Design review of the part built by this model. Coordinates are the model's own, in mm. A direction names the side the tool comes from. Round coordinates to 2 decimals unless told otherwise and drop trailing zeros. Write each loop counter-clockwise with the first axis right and the second up, starting at its lowest first coordinate (ties: lowest second). Pieces come first, ordered by that corner, then holes. Notation, with made-up numbers: (58, 82) -> (73, 82) arc R14 ccw to (73, 95) -> close; hole circle Ø8 at (-0.75, -11.75). An arc over 180 degrees is marked (long way). One line per question, with ' | ' between items. Start each with the question number.
1) For faces 1 (the flat face through (108.839, 0, 3)), 2 (the cylindrical face through (28.573, 0.209, 3.131)), 3 (the cylindrical face through (98.007, 1.411, 2.88)), list the 3-axis set-ups (+Z, -Z, +X, -X, +Y, -Y) from which the entire face can be reached by the end or side of a thin tool; tool diameter is ignored.
2) For probe 1 along Y at (x, z) = (-4.5, 1.5) (3 decimals); probe 2 along X at (y, z) = (2.5, 5); probe 3 along Y at (x, z) = (22, 2.25), list the stretches that pass through material, from the lowest coordinate up.
3) Insertion check: pin 1 Ø1 at (x, y) = (-29, 24.5) entering from -Z; pin 2 Ø3 at (x, y) = (101.5, -0.5) entering from -Z. Each pin has a flat end and moves straight along its axis. Give the tip position at first contact, or say it passes through.
4) Consider section B-B (z = 4.5). Give the boundary of the cut face in (x, y) (3 decimals).
5) Consider section A-A (y = 0). Give the boundary of the cut face in (x, z) (3 decimals), then the cut area to 3 significant figures.
```python
from build123d import *

# Parameters (mm, degrees)
SKETCH1_W               = 217.678
SKETCH1_H               = 63.5
BOSS_EXTRUDE1_DEPTH     = 6.35
CUT_EXTRUDE1_DEPTH      = 114.553128187
CUT_EXTRUDE1_DEPTH_BACK = 114.553128187
SKETCH3_R               = 4.699
CUT_EXTRUDE2_DEPTH      = 5.842


with BuildPart() as part:
    # Sketch1 → Boss-Extrude1 (new body)
    with BuildSketch(Plane.XY):
        Rectangle(SKETCH1_W, SKETCH1_H)
    extrude(amount=BOSS_EXTRUDE1_DEPTH)

    # Sketch2 → Cut-Extrude1 (cut, two sides: drawn at the far end of the back side and taken through both)
    with BuildSketch(Plane.XY.offset(6.35).offset(-CUT_EXTRUDE1_DEPTH_BACK)):
        with BuildLine():
            Line((19.05, -9.525), (-19.05, -9.525))
            ThreePointArc((-19.05, -9.525), (-28.575, 0), (-19.05, 9.525))
            Line((-19.05, 9.525), (19.05, 9.525))
            ThreePointArc((19.05, 9.525), (28.575, 0), (19.05, -9.525))
        make_face()
    extrude(amount=CUT_EXTRUDE1_DEPTH + CUT_EXTRUDE1_DEPTH_BACK, mode=Mode.SUBTRACT)

    # Sketch3 → Cut-Extrude2 (cut)
    with BuildSketch(Plane(origin=(0, 0, 0), x_dir=(-1, 0, 0), z_dir=(0, 0, -1))):
        with Locations((-102.489, 0)):
            Circle(SKETCH3_R)
        with Locations((102.489, 0)):
            Circle(SKETCH3_R)
    extrude(amount=-CUT_EXTRUDE2_DEPTH, mode=Mode.SUBTRACT)


solid = part.part
```
From the geometry:
1) face 1: +Z, -Z, +X, +Y, -Y | face 2: +Z, -Z | face 3: -Z
2) probe 1: y = -31.75 to -9.525, 9.525 to 31.75 | probe 2: x = -108.84 to -106.47, -98.51 to -28.24, 28.24 to 98.51, 106.47 to 108.84 | probe 3: y = -31.75 to -9.06, 9.06 to 31.75
3) pin 1: stops at z = 0 | pin 2: stops at z = 5.84
4) outline: (-108.839, -31.75) -> (108.839, -31.75) -> (108.839, 31.75) -> (-108.839, 31.75) -> close; hole circle Ø9.398 at (-102.489, 0); hole (-19.05, -9.525) -> (19.05, -9.525) arc R9.525 ccw to (19.05, 9.525) -> (-19.05, 9.525) arc R9.525 ccw to start; hole circle Ø9.398 at (102.489, 0)
5) outline: (-108.839, 0) -> (-107.188, 0) -> (-107.188, 5.842) -> (-97.79, 5.842) -> (-97.79, 0) -> (-28.575, 0) -> (-28.575, 6.35) -> (-108.839, 6.35) -> close; (28.575, 0) -> (97.79, 0) -> (97.79, 5.842) -> (107.188, 5.842) -> (107.188, 0) -> (108.839, 0) -> (108.839, 6.35) -> (28.575, 6.35) -> close | area: 910 mm2
